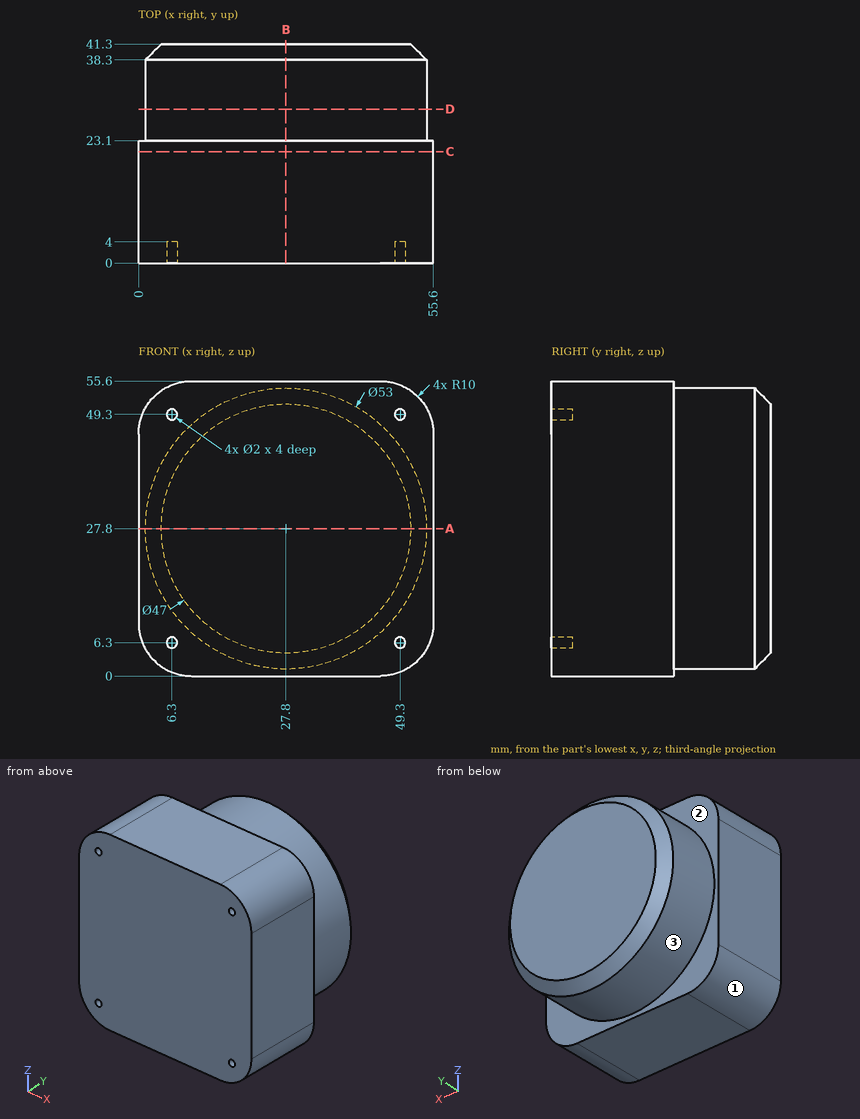
Verification items for this drawing (mm, ordinates from the low corner). Coordinates: 2 decimals unless noted, no trailing zeros. Order: outer loops, then holes, each group sorted by start corner. A loop starts at its lowest first (then second) coordinate and runs counter-clockwise, first axis right, second up. Notation, with made-up numbers: (14.25, 27) -> (44.25, 27) arc R17 cw to (44.25, 55) -> close; hole circle Ø4 at (-3.5, -29). An arc over 180 degrees is marked (long way). Answer as CSV lines item,"result". Start each with the question number.
1) Gauge pin test, flat ends, axial feed: pin 1 Ø10 at (x, y) = (17.5, 37) entering from +Z; pin 2 Ø1 at (x, z) = (6, 49) entering from -Y; pin 3 Ø1.5 at (x, y) = (48.5, 25) entering from -Z. Record the tip position at first contact, or that the pin passes through.
2) Release check for a two-part mould opening along X. For the marked faces 1, 2 and 3 record: released by +X, released by -X, zero draft, split by the parting line, or undercut.
3) Material ranges on L1, parallel to X at y = 1.8, z = 6.3; L2, parallel to X at y = 2, z = 6; L3, parallel to Z at x = 49, y = 1, recorded low to high. Write a range as [from, to].
4) Cross-section at D-D, the plane y = 29. Record the boundary of the cut face in (x, z), then the cut area to 3 significant figures.
5) Cross-section at C-C, the plane y = 21. Record the boundary of the cut face in (x, z).
6) Cross-section at A-A, the plane z = 27.8. Record the boundary of the cut face in (x, y).
7) Cross-section at B-B, the plane x = 27.8. Record the boundary of the cut face in (y, z), then the cut area to 3 significant figures.
Conclusion:
1,pin 1,"stops at z = 53.76"
1,pin 2,"stops at y = 4"
1,pin 3,"stops at z = 10.36"
2,face 1,"released by -X"
2,face 2,"zero draft"
2,face 3,"split by the parting line"
3,L1,"x = [0.71, 5.3], [7.3, 48.3], [50.3, 54.89]"
3,L2,"x = [0.83, 5.35], [7.25, 48.35], [50.25, 54.77]"
3,L3,"z = [0.6, 5.35], [7.25, 48.35], [50.25, 55]"
4,outline,"circle Ø53 at (27.8, 27.8)"
4,area,"2,210 mm²"
5,outline,"(0, 10) arc R10 ccw to (10, 0) -> (45.6, 0) arc R10 ccw to (55.6, 10) -> (55.6, 45.6) arc R10 ccw to (45.6, 55.6) -> (10, 55.6) arc R10 ccw to (0, 45.6) -> close"
6,outline,"(0, 0) -> (55.6, 0) -> (55.6, 23.1) -> (54.3, 23.1) -> (54.3, 38.3) -> (51.3, 41.3) -> (4.3, 41.3) -> (1.3, 38.3) -> (1.3, 23.1) -> (0, 23.1) -> close"
7,outline,"(0, 0) -> (23.1, 0) -> (23.1, 1.3) -> (38.3, 1.3) -> (41.3, 4.3) -> (41.3, 51.3) -> (38.3, 54.3) -> (23.1, 54.3) -> (23.1, 55.6) -> (0, 55.6) -> close"
7,area,"2,240 mm²"
